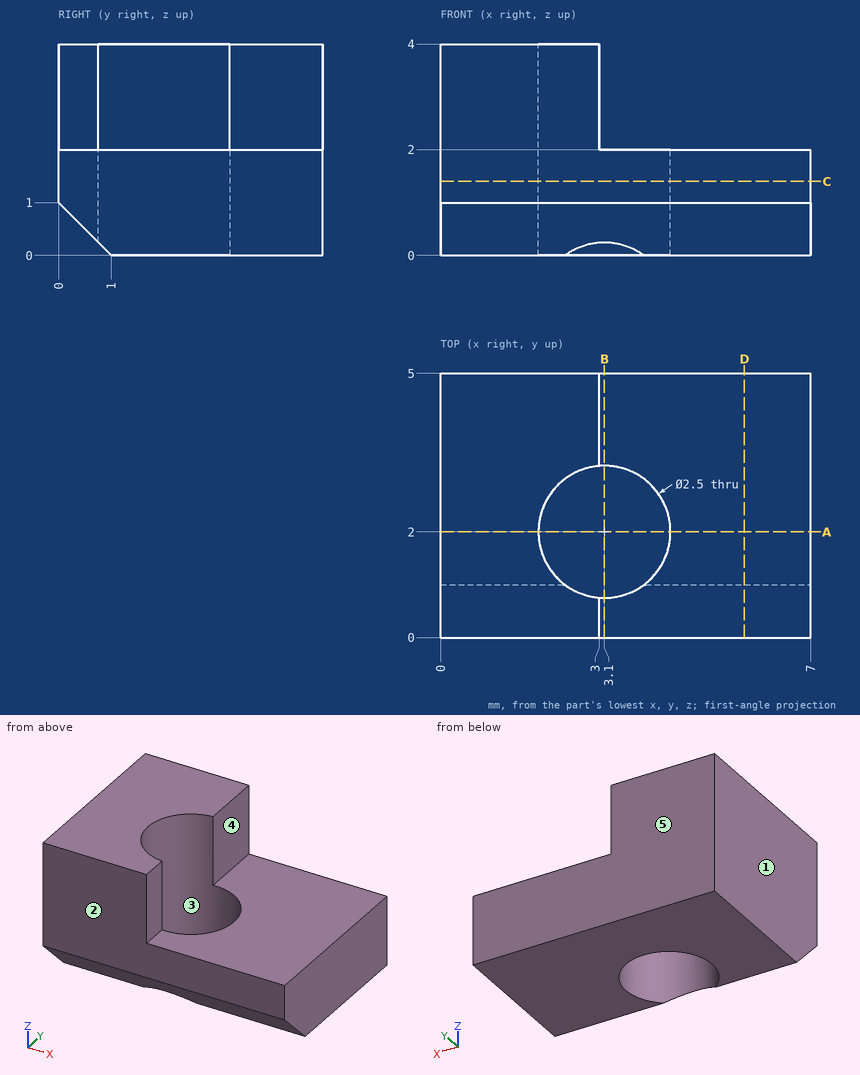
Design review of the part shown in the three views and the two pictorial views. Dimensions are in mm from the part's minimum x, y and z. A direction names the side the tool comes from. Give positions to 0.01 mm unless a question says otherwise; leave off trailing zeros. Loops run counter-clockwise (first coordinate to the right, second up) from the corner with the lowest first, then second, coordinate; pieces in that order, holes last. Notation, with made-up numbers: M 51,26.25 L 107,26.25 A21 cw 107,31.25 Z; hole C 34.25,62.25 d10. An arc over 180 degrees is marked long. Put each result on its own line as item: value. Start each with the question number.
(1) Add section A-A, the plane y = 2. Write out the cut boundary in (x, z).
(2) Wall thickness on L1, parallel to X at y = 2, z = 1.6; L2, parallel to Y at x = 3.1, z = 1.55; L3, parallel to X at y = 0.2, z = 2.6: over which ranges is each line inside the solid? List them lowest first.
(3) Add section B-B, the plane x = 3.1. Write out the cut boundary in (y, z).
(4) For pin 1 (0.9 mm diameter, centred on y = 4, z = 3.5, fed in from +X); pin 2 (1.2 mm diameter, centred on x = 5, y = 3, fed in from +Z), all flat-tipped, find the tip position at first contact; note any pin that passes through.
(5) The part is to be moulded in two halves that separate along Y. For the marked faces 1, 2 and 3, say which applies: +Y half, -Y half, draft (parallel to the pull), parting line (faces both ways), or undercut.
(6) Add section D-D, the plane x = 5.75. Write out the cut boundary in (y, z).
(7) Add section C-C, the plane z = 1.4. Write out the cut boundary in (x, y), then the cut area to 3 significant figures.
(8) Machinability: for the marked faces 4 and 5, which of the approach directions +Z, -Z, +X, -X, +Y, -Y give a long, thin tool a straight path to every point of the face, cutting with its end or side? Answer none if there is none.
Result:
1. outline: M 0,0 L 1.85,0 L 1.85,4 L 0,4 Z; M 4.35,0 L 7,0 L 7,2 L 4.35,2 Z
2. L1: x = 0 to 1.85, 4.35 to 7
2. L2: y = 0 to 0.75, 3.25 to 5
2. L3: x = 0 to 3
3. outline: M 0,1 L 0.75,0.25 L 0.75,2 L 0,2 Z; M 3.25,0 L 5,0 L 5,2 L 3.25,2 Z
4. pin 1: stops at x = 3
4. pin 2: stops at z = 2
5. face 1: draft
5. face 2: -Y half
5. face 3: undercut
6. outline: M 0,1 L 1,0 L 5,0 L 5,2 L 0,2 Z
7. outline: M 0,0 L 7,0 L 7,5 L 0,5 Z; hole C 3.1,2 d2.5
7. area: 30.1 mm^2
8. face 4: +Z, +X, +Y, -Y
8. face 5: +Z, -Z, +X, -X, +Y
